Geometry check sheet. Reference: the model listing, model coordinates, mm. Face numbers are marked on the shaded views. A direction names the side the tool comes from. Give positions to 0.01 mm unless a question says otherwise; leave off trailing zeros. Write each loop counter-clockwise with the first axis right and the second up, starting at its lowest first coordinate (ties: lowest second). Pieces come first, ordered by that corner, then holes. Notation, with made-up numbers: (81, 62) -> (138, 62) arc R31 ccw to (138, 97) -> close; hole circle Ø1 at (37, -37.5). An arc over 180 degrees is marked (long way). One line per item, written item: value.
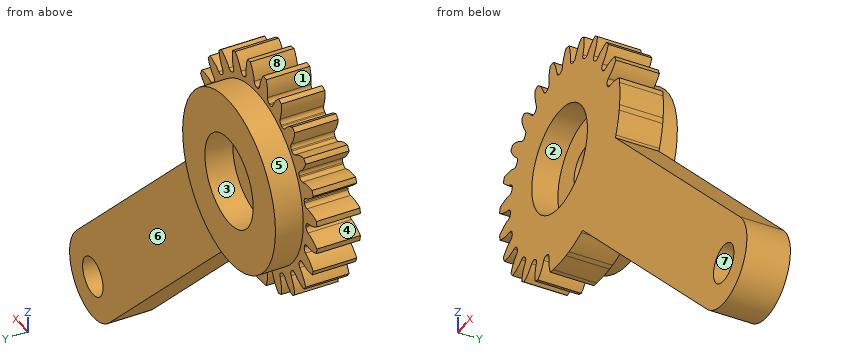
from build123d import *

# Parameters (mm, degrees)
SKETCH2_R                = 13
SKETCH2_R_2              = 5.2
BOSS_EXTRUDE1_DEPTH      = 5
CUT_EXTRUDE1_DEPTH       = 20.052558883
FILLET1_R                = 0.5
CIRPATTERN1_COUNT        = 24
FILLET1_OF_CIRPATTERN1_R = 0.5
EXTRUDE_START            = -5
EXTRUDE_1_OUTLINE_R      = 2.2
EXTRUDE_1_DEPTH          = 5
SKETCH_5_R               = 10
SKETCH_5_R_2             = 5.2
EXTRUDE_2_DEPTH          = 3.2
SKETCH_6_R               = 6
CUT_EXTRUDE_1_DEPTH      = 3
SKETCH_7_R               = 5.2
SKETCH_7_R_2             = 2.5
EXTRUDE_3_DEPTH          = 2


# Read off the part's stored shape, not the designer's step: 凸台-拉伸1
with BuildPart() as part:
    # Sketch2 → Boss-Extrude1 (new body)
    with BuildSketch(Plane(origin=(0, 0, 0), x_dir=(1, 0, 0), z_dir=(0, 1, 0))):
        with Locations(Location((0, 0, 0), (0, 0, 270))):
            Circle(SKETCH2_R)
        with Locations(Location((0, 0, 0), (0, 0, 270))):
            Circle(SKETCH2_R_2, mode=Mode.SUBTRACT)
    extrude(amount=BOSS_EXTRUDE1_DEPTH)

    # Sketch3 → Cut-Extrude1 (cut, through all)
    with BuildSketch(Plane(origin=(0, 5, 0), x_dir=(1, 0, 0), z_dir=(0, 1, 0))):
        with BuildLine():
            ThreePointArc((0.527459192, 10.586868602), (0, 10.6), (-0.527459192, 10.586868602))
            ThreePointArc((-0.527459192, 10.586868602), (-0.776880215, 11.820955553), (-1.379068427, 12.926645747))
            ThreePointArc((-1.379068427, 12.926645747), (0, 13), (1.379068427, 12.926645747))
            ThreePointArc((1.379068427, 12.926645747), (0.776880215, 11.820955553), (0.527459192, 10.586868602))
        make_face()
    cut_extrude1 = extrude(amount=-CUT_EXTRUDE1_DEPTH, mode=Mode.SUBTRACT)

    # Fillet1
    fillet1_edges = [part.edges().sort_by_distance(p)[0] for p in [
        (-0.527459192, 2.5, -10.586868602),
        (0.527459192, 2.5, -10.586868602),
    ]]
    fillet(fillet1_edges, radius=FILLET1_R)

    # CirPattern1: Cut-Extrude1 ×24 about axis
    cirpattern1_axis = Axis((0, 0, 0), (0, 1, 0))
    for i in range(1, CIRPATTERN1_COUNT):
        add(cut_extrude1.rotate(cirpattern1_axis, i * 360 / CIRPATTERN1_COUNT), mode=Mode.SUBTRACT)

    # Fillet1 of CirPattern1
    fillet1_of_cirpattern1_edges = [part.edges().sort_by_distance(p)[0] for p in [
        (-3.249569678, 2.5, -10.089613318),
        (-2.230596767, 2.5, -10.362646287),
        (-5.750227361, 2.5, -8.90476756),
        (-4.836641242, 2.5, -9.432226752),
        (-7.859016551, 2.5, -7.113076609),
        (-7.113076609, 2.5, -7.859016551),
        (-9.432226752, 2.5, -4.836641242),
        (-8.90476756, 2.5, -5.750227361),
        (-10.362646287, 2.5, -2.230596767),
        (-10.089613318, 2.5, -3.249569678),
        (-10.586868602, 2.5, 0.527459192),
        (-10.586868602, 2.5, -0.527459192),
        (-10.089613318, 2.5, 3.249569678),
        (-10.362646287, 2.5, 2.230596767),
        (-8.90476756, 2.5, 5.750227361),
        (-9.432226752, 2.5, 4.836641242),
        (-7.113076609, 2.5, 7.859016551),
        (-7.859016551, 2.5, 7.113076609),
        (-4.836641242, 2.5, 9.432226752),
        (-5.750227361, 2.5, 8.90476756),
        (-2.230596767, 2.5, 10.362646287),
        (-3.249569678, 2.5, 10.089613318),
        (0.527459192, 2.5, 10.586868602),
        (-0.527459192, 2.5, 10.586868602),
        (3.249569678, 2.5, 10.089613318),
        (2.230596767, 2.5, 10.362646287),
        (5.750227361, 2.5, 8.90476756),
        (4.836641242, 2.5, 9.432226752),
        (7.859016551, 2.5, 7.113076609),
        (7.113076609, 2.5, 7.859016551),
        (9.432226752, 2.5, 4.836641242),
        (8.90476756, 2.5, 5.750227361),
        (10.362646287, 2.5, 2.230596767),
        (10.089613318, 2.5, 3.249569678),
        (10.586868602, 2.5, -0.527459192),
        (10.586868602, 2.5, 0.527459192),
        (10.089613318, 2.5, -3.249569678),
        (10.362646287, 2.5, -2.230596767),
        (8.90476756, 2.5, -5.750227361),
        (9.432226752, 2.5, -4.836641242),
        (7.113076609, 2.5, -7.859016551),
        (7.859016551, 2.5, -7.113076609),
        (4.836641242, 2.5, -9.432226752),
        (5.750227361, 2.5, -8.90476756),
        (2.230596767, 2.5, -10.362646287),
        (3.249569678, 2.5, -10.089613318),
    ]]
    fillet(fillet1_of_cirpattern1_edges, radius=FILLET1_OF_CIRPATTERN1_R)

    # 凸台-拉伸1 outline → 凸台-拉伸1 (add)
    # profile 1 of 5: a face of its own
    with BuildSketch(Plane(origin=(0, 5, 0), x_dir=(1, 0, 0), z_dir=(0, 1, 0)).offset(EXTRUDE_START)):
        with BuildLine():
            ThreePointArc((12.926645747, -1.379068427), (13, 0), (12.926645747, 1.379068427))
            ThreePointArc((12.926645747, 1.379068427), (12.025072485, 0.857236447), (11.02318205, 0.572002303))
            ThreePointArc((11.02318205, 0.572002303), (10.718934665, 0.401929215), (10.599738984, 0.074387285))
            ThreePointArc((10.599738984, 0.074387285), (10.6, 0), (10.599738984, -0.074387285))
            ThreePointArc((10.599738984, -0.074387285), (10.718934665, -0.401929215), (11.02318205, -0.572002303))
            ThreePointArc((11.02318205, -0.572002303), (12.025072485, -0.857236447), (12.926645747, -1.379068427))
        make_face()
    # profile 2 of 5: a face of its own
    with BuildSketch(Plane(origin=(0, 5, 0), x_dir=(1, 0, 0), z_dir=(0, 1, 0)).offset(EXTRUDE_START)):
        with BuildLine():
            ThreePointArc((12.843110147, 2.013584299), (12.557035741, 3.364647587), (12.129251801, 4.677739919))
            ThreePointArc((12.129251801, 4.677739919), (11.393458958, 3.940344601), (10.49953114, 3.405521249))
            ThreePointArc((10.49953114, 3.405521249), (10.249668888, 3.162498244), (10.219308791, 2.815266922))
            ThreePointArc((10.219308791, 2.815266922), (10.238813759, 2.743481878), (10.257814483, 2.671561723))
            ThreePointArc((10.257814483, 2.671561723), (10.457722759, 2.386030625), (10.79562132, 2.300497655))
            ThreePointArc((10.79562132, 2.300497655), (11.837197196, 2.284290955), (12.843110147, 2.013584299))
        make_face()
    # profile 3 of 5: a face of its own
    with BuildSketch(Plane(origin=(0, 5, 0), x_dir=(1, 0, 0), z_dir=(0, 1, 0)).offset(EXTRUDE_START)):
        with BuildLine():
            ThreePointArc((11.884337816, 5.269014582), (11.9536425, 5.109836689), (12.020815281, 4.949747468))
            Line((12.020815281, 4.949747468), (38.890872965, 31.819805153))
            ThreePointArc((38.890872965, 31.819805153), (38.890872965, 38.890872965), (31.819805153, 38.890872965))
            Line((31.819805153, 38.890872965), (4.949747468, 12.020815281))
            ThreePointArc((4.949747468, 12.020815281), (5.109836689, 11.9536425), (5.269014582, 11.884337816))
            ThreePointArc((5.269014582, 11.884337816), (5.270147703, 10.842636478), (5.0162225, 9.832356838))
            ThreePointArc((5.0162225, 9.832356838), (5.011386422, 9.483834329), (5.235448214, 9.216836876))
            ThreePointArc((5.235448214, 9.216836876), (5.3, 9.17986928), (5.364290771, 9.142449591))
            ThreePointArc((5.364290771, 9.142449591), (5.707548244, 9.081905114), (6.006959551, 9.260354535))
            ThreePointArc((6.006959551, 9.260354535), (6.754924783, 9.985400031), (7.657631165, 10.505269389))
            ThreePointArc((7.657631165, 10.505269389), (7.913898577, 10.313593424), (8.165370229, 10.115667502))
            ThreePointArc((8.165370229, 10.115667502), (7.896852594, 9.109168003), (7.390100071, 8.199033485))
            ThreePointArc((7.390100071, 8.199033485), (7.295224515, 7.863638262), (7.442547561, 7.547747068))
            ThreePointArc((7.442547561, 7.547747068), (7.495331881, 7.495331881), (7.547747068, 7.442547561))
            ThreePointArc((7.547747068, 7.442547561), (7.863638262, 7.295224515), (8.199033485, 7.390100071))
            ThreePointArc((8.199033485, 7.390100071), (9.109168003, 7.896852594), (10.115667502, 8.165370229))
            ThreePointArc((10.115667502, 8.165370229), (10.313593424, 7.913898577), (10.505269389, 7.657631165))
            ThreePointArc((10.505269389, 7.657631165), (9.985400031, 6.754924783), (9.260354535, 6.006959551))
            ThreePointArc((9.260354535, 6.006959551), (9.081905114, 5.707548244), (9.142449591, 5.364290771))
            ThreePointArc((9.142449591, 5.364290771), (9.17986928, 5.3), (9.216836876, 5.235448214))
            ThreePointArc((9.216836876, 5.235448214), (9.483834329, 5.011386422), (9.832356838, 5.0162225))
            ThreePointArc((9.832356838, 5.0162225), (10.842636478, 5.270147703), (11.884337816, 5.269014582))
        make_face()
        with Locations((35.355339059, 35.355339059)):
            Circle(EXTRUDE_1_OUTLINE_R, mode=Mode.SUBTRACT)
    # profile 4 of 5: a face of its own
    with BuildSketch(Plane(origin=(0, 5, 0), x_dir=(1, 0, 0), z_dir=(0, 1, 0)).offset(EXTRUDE_START)):
        with BuildLine():
            ThreePointArc((0.572002303, 11.02318205), (0.857236447, 12.025072485), (1.379068427, 12.926645747))
            ThreePointArc((1.379068427, 12.926645747), (0, 13), (-1.379068427, 12.926645747))
            ThreePointArc((-1.379068427, 12.926645747), (-0.857236447, 12.025072485), (-0.572002303, 11.02318205))
            ThreePointArc((-0.572002303, 11.02318205), (-0.401929215, 10.718934665), (-0.074387285, 10.599738984))
            ThreePointArc((-0.074387285, 10.599738984), (0, 10.6), (0.074387285, 10.599738984))
            ThreePointArc((0.074387285, 10.599738984), (0.401929215, 10.718934665), (0.572002303, 11.02318205))
        make_face()
    # profile 5 of 5: a face of its own
    with BuildSketch(Plane(origin=(0, 5, 0), x_dir=(1, 0, 0), z_dir=(0, 1, 0)).offset(EXTRUDE_START)):
        with BuildLine():
            ThreePointArc((3.405521249, 10.49953114), (3.940344601, 11.393458958), (4.677739919, 12.129251801))
            ThreePointArc((4.677739919, 12.129251801), (3.364647587, 12.557035741), (2.013584299, 12.843110147))
            ThreePointArc((2.013584299, 12.843110147), (2.284290955, 11.837197196), (2.300497655, 10.79562132))
            ThreePointArc((2.300497655, 10.79562132), (2.386030625, 10.457722759), (2.671561723, 10.257814483))
            ThreePointArc((2.671561723, 10.257814483), (2.743481878, 10.238813759), (2.815266922, 10.219308791))
            ThreePointArc((2.815266922, 10.219308791), (3.162498244, 10.249668888), (3.405521249, 10.49953114))
        make_face()
    extrude(amount=EXTRUDE_1_DEPTH)

    # 草图5 → 凸台-拉伸2 (add)
    with BuildSketch(Plane(origin=(0, 5, 0), x_dir=(1, 0, 0), z_dir=(0, 1, 0))):
        with Locations(Location((0, 0, 0), (0, 0, 270))):
            Circle(SKETCH_5_R)
        with Locations(Location((0, 0, 0), (0, 0, 270))):
            Circle(SKETCH_5_R_2, mode=Mode.SUBTRACT)
    extrude(amount=EXTRUDE_2_DEPTH)

    # 草图6 → 切除-拉伸1 (cut)
    with BuildSketch(Plane.XZ):
        with Locations(Location((0, 0, 0), (0, 0, 270))):
            Circle(SKETCH_6_R)
    extrude(amount=-CUT_EXTRUDE_1_DEPTH, mode=Mode.SUBTRACT)

    # 草图7 → 凸台-拉伸3 (add)
    with BuildSketch(Plane.XZ.offset(-3)):
        with Locations(Location((0, 0, 0), (0, 0, 270))):
            Circle(SKETCH_7_R)
        with Locations(Location((0, 0, 0), (0, 0, 270))):
            Circle(SKETCH_7_R_2, mode=Mode.SUBTRACT)
    extrude(amount=-EXTRUDE_3_DEPTH)


solid = part.part
1) Sectioned sample at C-C on x = 20. Record the cut outline in (y, z), plus the area to 3 significant figures.
Verdict:
outline: (0, -27.07) -> (5, -27.07) -> (5, -12.93) -> (0, -12.93) -> close
area: 70.7 mm^2
2) Scan lines: probe 1 along X at (y, z) = (6.2, 0); probe 2 along Z at (x, y) = (8, 7.5); probe 3 along Y at (x, z) = (10, -3.5). Record each from-to range of solid material in increasing order.
Verdict:
probe 1: -10 to -5.2, 5.2 to 10
probe 2: -6 to 6
probe 3: 0 to 5
3) Mould release check, pull along X, two halves, no side actions. Record for the marked faces 5, 6, 7 and 8: released by +X, released by -X, zero draft, split by the parting line, or undercut.
Verdict:
face 5: split by the parting line
face 6: zero draft
face 7: undercut
face 8: undercut
4) Sectioned sample at B-B on y = 1.75. Give the number of separate pieces and of enclosed holes in the cut face, plus the area to 3 significant figures.
Verdict:
separate pieces: 1
enclosed holes: 2
area: 749 mm^2
5) Tool access check on the marked faces 1, 2, 3 and 4. Record the directions out of +Z, -Z, +X, -X, +Y, -Y that give a thin tool (end or side, any length) a straight path to the whole face; none if there is none.
Verdict:
face 1: +Y, -Y
face 2: -Y
face 3: +Y
face 4: -X, +Y, -Y
6) Depth check by flat-ended pin: pin 1 Ø12 at (x, z) = (24.5, -20) entering from +Y; pin 2 Ø11 at (x, z) = (0, 0) entering from -Y; pin 3 Ø1.5 at (x, y) = (15.5, 1.5) entering from -Z. Enter the tip coordinate at first touch or a pass-through.
Verdict:
pin 1: y = 5
pin 2: y = 3
pin 3: z = -23.32
7) Sectioned sample at A-A on y = 6. Record the cut outline in (x, z).
Verdict:
outline: circle Ø20 at (0, 0); hole circle Ø10.4 at (0, 0)
